Input: dimensioned drawing with shaded views. Units: mm. Origin: part minimum x, y, z. Round coordinates to 2 decimals unless told otherwise and drop trailing zeros. Write each loop counter-clockwise with the first axis right and the second up, starting at its lowest first coordinate (ties: lowest second). Pieces come first, ordered by that corner, then holes. Notation, with made-up numbers: M 34.5,-5 L 90.5,-5 A21 cw 90.5,-1 Z; hole C 32,43.5 d1. An arc over 180 degrees is marked long. Answer in a Markdown table with one row per item. Add a question column.
Item 1: Cut plane A-A on x = 76.2. Give the number of separate pieces and of enclosed holes in the cut face, and give its area (3 significant figures).
Item 2: Contact query for flat-ended pins moving along their axis: pin 1 (2 mm diameter, centred on y = 0.5, z = 52.5, fed in from +X); pin 2 (2 mm diameter, centred on x = 69.5, y = 1.5, fed in from +Z); pin 3 (0.8 mm diameter, centred on y = 1, z = 82, fed in from -X); pin 4 (5.5 mm diameter, centred on x = 76.2, z = 12.7, fed in from +Y). Output: stop coordinate, or through.
Item 3: Cut plane D-D on x = 124.5. Return loops of the section in (y, z).
Item 4: Material intervals for probe 1 along Z at (x, y) = (76.2, 5) (1 decimal); probe 2 along X at (y, z) = (3.25, 54.5); probe 3 along X at (y, z) = (4.5, 12), sorted ascending.
Item 5: Cut plane B-B on z = 68. Return loops of the section in (x, y), and give its area (3 significant figures).
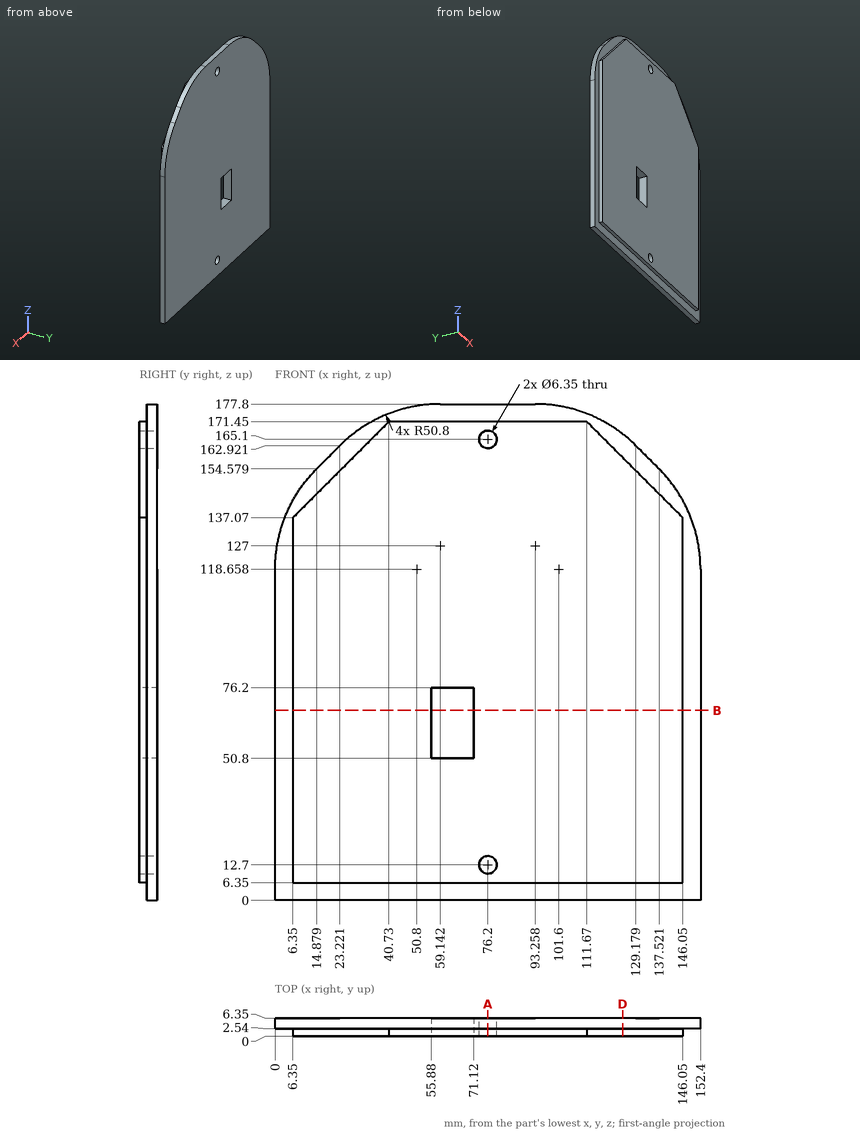
Results below:
| question | item | result |
|---|---|---|
| 1 | separate pieces | 3 |
| 1 | enclosed holes | 0 |
| 1 | area | 1,020 mm2 |
| 2 | pin 1 | x = 146.05 |
| 2 | pin 2 | z = 171.45 |
| 2 | pin 3 | x = 6.35 |
| 2 | pin 4 | through |
| 3 | outline | M 0,6.35 L 2.54,6.35 L 2.54,0 L 6.35,0 L 6.35,167.06 L 2.54,167.06 L 2.54,158.62 L 0,158.62 Z |
| 4 | probe 1 | 0 to 9.5, 15.9 to 161.9, 168.3 to 177.8 |
| 4 | probe 2 | 0 to 55.88, 71.12 to 152.4 |
| 4 | probe 3 | 0 to 73.1, 79.3 to 152.4 |
| 5 | outline | M 0,2.54 L 6.35,2.54 L 6.35,0 L 55.88,0 L 55.88,6.35 L 0,6.35 Z; M 71.12,0 L 146.05,0 L 146.05,2.54 L 152.4,2.54 L 152.4,6.35 L 71.12,6.35 Z |
| 5 | area | 839 mm2 |
